Could you check a few things on this model? Use its own coordinates, in mm. A direction names the side the tool comes from. Give positions to 0.01 mm unless a question says otherwise; leave off trailing zeros. Write each loop counter-clockwise with the first axis right and the second up, starting at its lowest first coordinate (ties: lowest second). Pieces come first, ordered by that corner, then holes. Notation, with made-up numbers: (39.5, 1) -> (76.5, 1) arc R28 ccw to (76.5, 40) -> close; hole circle Ø8 at (53, 73.25). An arc over 180 degrees is marked (long way). Write item = value, one per line. Start each with the question number.
```python
from build123d import *

# Parameters (mm, degrees)
BOSS_EXTRUDE1_DEPTH   = 25.4
M10_CLEARANCE_HOLE1_D = 12
M10_CLEARANCE_HOLE2_D = 12
FILLET1_R             = 30.32


with BuildPart() as part:
    # Sketch1 → Boss-Extrude1 (new body)
    with BuildSketch(Plane.XY):
        Polygon((0, 194.731808123), (0, -59.268191877), (-127, -59.268191877), (-127, -8.468191877), (-50.8, -8.468191877), (-50.8, 194.731808123), align=None)
    extrude(amount=BOSS_EXTRUDE1_DEPTH)

    # M10 Clearance Hole1 (through all)
    with Locations(Plane(origin=(0, -8.468191877, 0), x_dir=(1, 0, 0), z_dir=(0, 1, 0))):
        with Locations((-114.3, -12.7), (-88.9, -12.7)):
            Hole(M10_CLEARANCE_HOLE1_D / 2)

    # M10 Clearance Hole2 (through all)
    with Locations(Plane.ZY.offset(50.8)):
        with Locations((12.7, 169.331808123), (12.7, 105.831808123)):
            Hole(M10_CLEARANCE_HOLE2_D / 2)

    # Fillet1
    fillet1_edges = [part.edges().sort_by_distance(p)[0] for p in [
        (-50.8, -8.468191877, 12.7),
    ]]
    fillet(fillet1_edges, radius=FILLET1_R)


solid = part.part
```
(1) Imagine slicing it at D-D (y = 83.5). Please give me the cut outline in (x, z), then the cut area to 3 significant figures.
(2) We'd pull the mould along X, two halves only. Please class faces 1 (the flat face through (-50.8, 107, 21)), 2 (the flat face through (-34, 41, 25.4)), 3 (the cylindrical face through (-120.023, -34.224, 10.898)), 4 (the cylindrical face through (-82.906, -34.224, 12.436)): released by +X, released by -X, zero draft, split by the parting line, or undercut.
(3) Imagine slicing it at C-C (x = -40.5). Please give me the cut outline in (y, z).
(4) If I drill on line 1 along Y through (x, z) = (-11.5, 12.7); line 2 along Z through (x, y) = (-114.3, -33); line 3 along Y through (x, z) = (-27, 17.25), over which ranges is the centre line in solid material (lowest first)? Write a range as from..to.
(5) On a 3-axis mill with a long thin cutter (end or side, diameter ignored), from which of +Z, -Z, +X, -X, +Y, -Y can I reach the whole of each face in a straight line? I mean faces 5 (the flat face through (0, 70, 13)), 6 (the flat face through (-104, -8.468, 13)). Say none if no direction works.
(6) I'm going to push flat-ended pins straight in: pin 1 (12 mm diameter, centred on y = 85.5, z = 12, fed in from -X); pin 2 (1.5 mm diameter, centred on x = -72.5, z = 18, fed in from +Y); pin 3 (7.5 mm diameter, centred on x = -105.5, z = 10.5, fed in from +Y). Where does each tip first touch, or does it pass through?
(7) Imagine slicing it at B-B (z = 12.7). Please give me the cut outline in (x, y), then the cut area to 3 significant figures.
(8) Imagine slicing it at A-A (x = -114.3). Please give me the cut outline in (y, z), then the cut area to 3 significant figures.
Answers below:
q1.outline = (-50.8, 0) -> (0, 0) -> (0, 25.4) -> (-50.8, 25.4) -> close
q1.area = 1,290 mm^2
q2.face_1 = released by -X
q2.face_2 = zero draft
q2.face_3 = undercut
q2.face_4 = undercut
q3.outline = (-59.27, 0) -> (194.73, 0) -> (194.73, 25.4) -> (-59.27, 25.4) -> close; hole circle Ø12 at (105.83, 12.7); hole circle Ø12 at (169.33, 12.7)
q4.line_1 = -59.27..99.83, 111.83..163.33, 175.33..194.73
q4.line_2 = 0..6.7, 18.7..25.4
q4.line_3 = -59.27..101.92, 109.74..165.42, 173.24..194.73
q5.face_5 = +Z, -Z, +X, +Y, -Y
q5.face_6 = +Z, -Z, -X, +Y
q6.pin_1 = -50.8
q6.pin_2 = -6.98
q6.pin_3 = -8.47
q7.outline = (-127, -59.27) -> (-120.3, -59.27) -> (-120.3, -8.47) -> (-127, -8.47) -> close; (-108.3, -59.27) -> (-94.9, -59.27) -> (-94.9, -8.47) -> (-108.3, -8.47) -> close; (-82.9, -59.27) -> (0, -59.27) -> (0, 99.83) -> (-50.8, 99.83) -> (-50.8, 21.85) arc R30.32 cw to (-81.12, -8.47) -> (-82.9, -8.47) -> close; (-50.8, 111.83) -> (0, 111.83) -> (0, 163.33) -> (-50.8, 163.33) -> close; (-50.8, 175.33) -> (0, 175.33) -> (0, 194.73) -> (-50.8, 194.73) -> close
q7.area = 14,500 mm^2
q8.outline = (-59.27, 0) -> (-8.47, 0) -> (-8.47, 6.7) -> (-59.27, 6.7) -> close; (-59.27, 18.7) -> (-8.47, 18.7) -> (-8.47, 25.4) -> (-59.27, 25.4) -> close
q8.area = 681 mm^2
